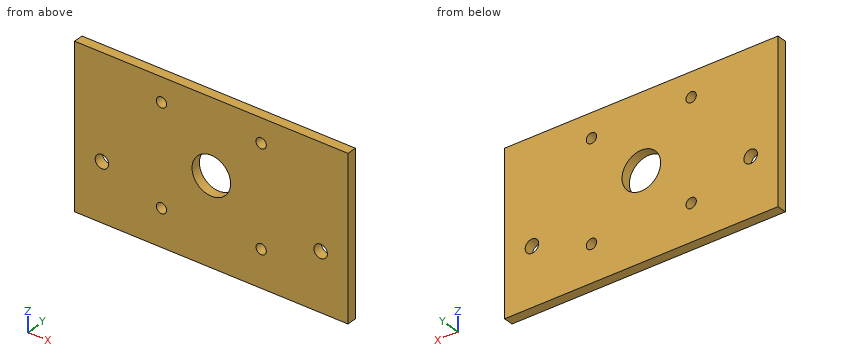
```python
from build123d import *

# Parameters (mm, degrees)
SKETCH1_W           = 130
SKETCH1_H           = 90
BOSS_EXTRUDE1_DEPTH = 3
SKETCH2_R           = 1.6
CUT_EXTRUDE1_DEPTH  = 10
SKETCH3_R           = 2.1
CUT_EXTRUDE2_DEPTH  = 10
SKETCH4_R           = 6
CUT_EXTRUDE3_DEPTH  = 10
SKETCH5_W           = 211.899285322
SKETCH5_H           = 138.032985156
SKETCH5_W_2         = 85
SKETCH5_H_2         = 50
CUT_EXTRUDE4_DEPTH  = 10


with BuildPart() as part:
    # Sketch1 → Boss-Extrude1 (new body)
    with BuildSketch(Plane(origin=(0, 0, 0), x_dir=(1, 0, 0), z_dir=(0, 1, 0))):
        Rectangle(SKETCH1_W, SKETCH1_H)
    extrude(amount=BOSS_EXTRUDE1_DEPTH)

    # Sketch2 → Cut-Extrude1 (cut)
    with BuildSketch(Plane(origin=(0, 3, 0), x_dir=(1, 0, 0), z_dir=(0, 1, 0))):
        with Locations(Location((15.5, 2.5, 0), (0, 0, 270))):
            Circle(SKETCH2_R)
        with Locations(Location((-15.5, 2.5, 0), (0, 0, 270))):
            Circle(SKETCH2_R)
        with Locations(Location((-15.5, 33.5, 0), (0, 0, 270))):
            Circle(SKETCH2_R)
        with Locations(Location((15.5, 33.5, 0), (0, 0, 270))):
            Circle(SKETCH2_R)
    extrude(amount=-CUT_EXTRUDE1_DEPTH, mode=Mode.SUBTRACT)

    # Sketch3 → Cut-Extrude2 (cut)
    with BuildSketch(Plane.XZ):
        with Locations(Location((-34, -27, 0), (0, 0, 270))):
            Circle(SKETCH3_R)
        with Locations(Location((34, -27, 0), (0, 0, 270))):
            Circle(SKETCH3_R)
    extrude(amount=-CUT_EXTRUDE2_DEPTH, mode=Mode.SUBTRACT)

    # Sketch4 → Cut-Extrude3 (cut)
    with BuildSketch(Plane.XZ):
        with Locations(Location((0, -18, 0), (0, 0, 270))):
            Circle(SKETCH4_R)
    extrude(amount=-CUT_EXTRUDE3_DEPTH, mode=Mode.SUBTRACT)

    # Sketch5 → Cut-Extrude4 (cut)
    with BuildSketch(Plane(origin=(0, 3, 0), x_dir=(1, 0, 0), z_dir=(0, 1, 0))):
        with Locations((0.497416163, -6.590764156)):
            Rectangle(SKETCH5_W, SKETCH5_H)
        with Locations((0, 20)):
            Rectangle(SKETCH5_W_2, SKETCH5_H_2, mode=Mode.SUBTRACT)
    extrude(amount=-CUT_EXTRUDE4_DEPTH, mode=Mode.SUBTRACT)


solid = part.part
```
Design review of the part built by this model. Coordinates are the model's own, in mm. Coordinates: 2 decimals unless noted, no trailing zeros. Loops run counter-clockwise (first coordinate to the right, second up) from the corner with the lowest first, then second, coordinate; pieces in that order, holes last. Notation, with made-up numbers: (-12.5, -26) -> (32.5, -26) arc R27 ccw to (32.5, 7) -> close; hole circle Ø9 at (-22.5, -0.75). An arc over 180 degrees is marked (long way). Answer as a JSON object with one key per item and string values.
Q1. To check wall thickness, follow L1, parallel to X at y = 1.15, z = -27; L2, parallel to X at y = 2.5, z = -26.5; L3, parallel to X at y = 2.35, z = -18. State the ranges of each line that lie inside material, in increasing order.
Answer block:
{"L1": "x = -42.5 to -36.1, -31.9 to 31.9, 36.1 to 42.5", "L2": "x = -42.5 to -36.04, -31.96 to 31.96, 36.04 to 42.5", "L3": "x = -42.5 to -6, 6 to 42.5"}
Q2. Take a section at C-C on y = 1.15. Give the boundary of the cut face in (x, z).
Answer block:
{"outline": "(-42.5, -45) -> (42.5, -45) -> (42.5, 5) -> (-42.5, 5) -> close; hole circle Ø4.2 at (-34, -27); hole circle Ø3.2 at (-15.5, -33.5); hole circle Ø3.2 at (-15.5, -2.5); hole circle Ø12 at (0, -18); hole circle Ø3.2 at (15.5, -33.5); hole circle Ø3.2 at (15.5, -2.5); hole circle Ø4.2 at (34, -27)"}
Q3. Take a section at D-D on x = -15.5. Give the boundary of the cut face in (y, z), plus the area to 3 significant figures.
Answer block:
{"outline": "(0, -45) -> (3, -45) -> (3, -35.1) -> (0, -35.1) -> close; (0, -31.9) -> (3, -31.9) -> (3, -4.1) -> (0, -4.1) -> close; (0, -0.9) -> (3, -0.9) -> (3, 5) -> (0, 5) -> close", "area": "131 mm^2"}
Q4. Take a section at B-B on x = 34. Give the boundary of the cut face in (y, z), plus the area to 3 significant figures.
Answer block:
{"outline": "(0, -45) -> (3, -45) -> (3, -29.1) -> (0, -29.1) -> close; (0, -24.9) -> (3, -24.9) -> (3, 5) -> (0, 5) -> close", "area": "137 mm^2"}
Q5. Take a section at A-A on z = -27. Give the boundary of the cut face in (x, y), plus the area to 3 significant figures.
Answer block:
{"outline": "(-42.5, 0) -> (-36.1, 0) -> (-36.1, 3) -> (-42.5, 3) -> close; (-31.9, 0) -> (31.9, 0) -> (31.9, 3) -> (-31.9, 3) -> close; (36.1, 0) -> (42.5, 0) -> (42.5, 3) -> (36.1, 3) -> close", "area": "230 mm^2"}
Q6. Clearance check with a flat-ended pin moving along its axis: pin 1 Ø4 at (x, z) = (15.5, -2.5) entering from -Y. State where the tip first meets the part, or that it passes through.
Answer block:
{"pin 1": "stops at y = 0"}
